```python
from build123d import *

# Parameters (mm, degrees)
SKETCH1_W           = 250
SKETCH1_H           = 150
SKETCH1_R           = 5
SKETCH1_W_2         = 40
SKETCH1_H_2         = 5
BOSS_EXTRUDE1_DEPTH = 10
SKETCH1_5_W         = 10
SKETCH1_5_H         = 150
BOSS_EXTRUDE2_DEPTH = 40
SKETCH1_6_R         = 5
BOSS_EXTRUDE3_DEPTH = 30
SKETCH1_7_W         = 40
SKETCH1_7_H         = 5
BOSS_EXTRUDE4_DEPTH = 30
SKETCH6_W           = 5
SKETCH6_H           = 20
SKETCH6_W_2         = 10
SKETCH6_H_2         = 20.218770798
BOSS_EXTRUDE5_DEPTH = 40
SKETCH7_W           = 5
SKETCH7_H           = 20
CUT_EXTRUDE1_DEPTH  = 10


with BuildPart() as part:
    # Sketch1 → Boss-Extrude1 (new body)
    with BuildSketch(Plane.XY):
        Rectangle(SKETCH1_W, SKETCH1_H)
        with Locations((-40, 0)):
            Circle(SKETCH1_R, mode=Mode.SUBTRACT)
        with Locations((60, -12.5)):
            Rectangle(SKETCH1_W_2, SKETCH1_H_2, mode=Mode.SUBTRACT)
        with Locations((60, 12.5)):
            Rectangle(SKETCH1_W_2, SKETCH1_H_2, mode=Mode.SUBTRACT)
    extrude(amount=BOSS_EXTRUDE1_DEPTH)

    # Sketch1<5> → Boss-Extrude2 (add)
    with BuildSketch(Plane.XY):
        with Locations((120, 0)):
            Rectangle(SKETCH1_5_W, SKETCH1_5_H)
    extrude(amount=BOSS_EXTRUDE2_DEPTH)

    # Sketch1<6> → Boss-Extrude3 (add)
    with BuildSketch(Plane.XY):
        with Locations((-40, 0)):
            Circle(SKETCH1_6_R)
    extrude(amount=BOSS_EXTRUDE3_DEPTH)

    # Sketch1<7> → Boss-Extrude4 (add)
    with BuildSketch(Plane.XY):
        with Locations((60, -12.5)):
            Rectangle(SKETCH1_7_W, SKETCH1_7_H)
        with Locations((60, 12.5)):
            Rectangle(SKETCH1_7_W, SKETCH1_7_H)
    extrude(amount=BOSS_EXTRUDE4_DEPTH)

    # Sketch6 → Boss-Extrude5 (add)
    with BuildSketch(Plane.ZY.offset(-40)):
        with Locations((12.5, 0)):
            Rectangle(SKETCH6_W, SKETCH6_H)
        with Locations((25, -0.109385399)):
            Rectangle(SKETCH6_W_2, SKETCH6_H_2)
    extrude(amount=-BOSS_EXTRUDE5_DEPTH)

    # Sketch7 → Cut-Extrude1 (cut)
    with BuildSketch(Plane.ZY.offset(-115)):
        with Locations((17.5, 0)):
            Rectangle(SKETCH7_W, SKETCH7_H)
    extrude(amount=-CUT_EXTRUDE1_DEPTH, mode=Mode.SUBTRACT)


solid = part.part
```
Part model, mm, in its own coordinate system. A direction names the side the tool comes from. Round coordinates to 2 decimals unless told otherwise and drop trailing zeros. Order: outer loops, then holes, each group sorted by start corner. A loop starts at its lowest first (then second) coordinate and runs counter-clockwise, first axis right, second up. Notation, with made-up numbers: M 0.5,3.25 L 51.5,3.25 A23 ccw 51.5,14.25 Z; hole C 70.5,74.25 d10. An arc over 180 degrees is marked long. Put each result on its own line as item: value. Start each with the question number.
1. Drop flat-ended pins along their axis: pin 1 (1.5 mm diameter, centred on x = -61, y = 16, fed in from +Z); pin 2 (24 mm diameter, centred on x = 53.5, y = 4.5, fed in from +Z); pin 3 (10 mm diameter, centred on x = 57.5, z = 24.5, fed in from +Y). Give the stop position or say it passes through.
2. Two-plate mould, pull along X, no slides. Class faces 1 (the face through (-125, -1, 5)), 2 (the face through (125, -1, 24)), 3 (the face through (60, -15, 20)), 4 (the face through (80, 0, 22)): +X half, -X half, draft (parallel to the pull), parting line (faces both ways), or undercut.
3. Drill centre lines: probe 1 along X at (y, z) = (-12.5, 24.5); probe 2 along X at (y, z) = (63, 37); probe 3 along Z at (x, y) = (-42.5, 21). Where is each one in solid material? Low to high. Write a range as [from, to].
4. Tool access for faces 5 (the face through (-40, 0, 30)), 6 (the face through (120, 0, 15)), 7 (the face through (120, 10, 17)), 8 (the face through (40, 0, 22)), 9 (the face through (-45, 0, 20)): list every direction of +Z, -Z, +X, -X, +Y, -Y with a clear straight run to the whole face (end or side of a thin tool).
5. Slice it at C-C on x = -40. List the corners of the cut face in (y, z), then the cut area to 3 significant figures.
6. Slice it at A-A on y = 0. List the corners of the cut face in (x, z).
7. Slice it at B-B on x = 66. List the corners of the cut face in (y, z), then the cut area to 3 significant figures.
8. Slice it at D-D on y = -55. List the corners of the cut face in (x, z), then the cut area to 3 significant figures.
Findings:
1. pin 1: z = 10
1. pin 2: z = 30
1. pin 3: y = 15
2. face 1: -X half
2. face 2: +X half
2. face 3: draft
2. face 4: undercut
3. probe 1: [40, 80], [115, 125]
3. probe 2: [115, 125]
3. probe 3: [0, 10]
4. face 5: +Z, -X, +Y, -Y
4. face 6: +X
4. face 7: +X, -X
4. face 8: +Z, +Y, -Y
4. face 9: +Z
5. outline: M -75,0 L 75,0 L 75,10 L 5,10 L 5,30 L -5,30 L -5,10 L -75,10 Z
5. area: 1,700 mm2
6. outline: M -125,0 L 125,0 L 125,15 L 115,15 L 115,10 L 80,10 L 80,15 L 40,15 L 40,10 L -35,10 L -35,30 L -45,30 L -45,10 L -125,10 Z; M 40,20 L 80,20 L 80,30 L 40,30 Z; M 115,20 L 125,20 L 125,40 L 115,40 Z
7. outline: M -75,0 L 75,0 L 75,10 L 15,10 L 15,30 L -15,30 L -15,10 L -75,10 Z; hole M -10,15 L 10,15 L 10,20 L -10,20 Z
7. area: 2,000 mm2
8. outline: M -125,0 L 125,0 L 125,40 L 115,40 L 115,10 L -125,10 Z
8. area: 2,800 mm2
